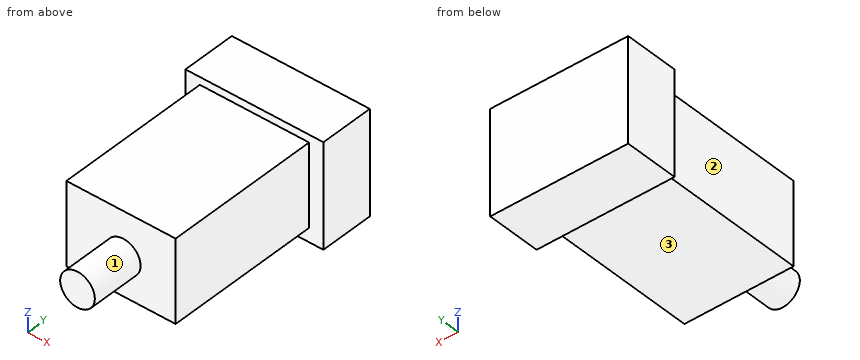
```python
from build123d import *

# Parameters (mm, degrees)
F0_W     = 101.638708
F0_H     = 76.456577
F1_DEPTH = 39.878
F2_W     = 80.470148
F2_H     = 60.710575
F3_DEPTH = 114.808
F4_R     = 12.763073
F5_DEPTH = 39.37
F6_W     = 52.336872
F6_H     = 92.136786
F7_DEPTH = 27.94


with BuildPart() as f1:
    # F0 (on Front) → F1 (new body)
    with BuildSketch(Plane.XZ):
        with Locations((-1.668697, -0.151697)):
            Rectangle(F0_W, F0_H)
    extrude(amount=F1_DEPTH)

    # F2 (on face) → F3 (join)
    with BuildSketch(Plane.XZ.offset(39.878)):
        with Locations((-1.668697, 2.139264)):
            Rectangle(F2_W, F2_H)
    extrude(amount=F3_DEPTH)

    # F4 (on face) → F5 (join)
    with BuildSketch(Plane.XZ.offset(154.686)):
        Circle(F4_R)
    extrude(amount=F5_DEPTH)

    # F6 (on face) → F7 (join)
    with BuildSketch(Plane.XY.offset(32.494552)):
        with Locations((-0.389457, -95.996715)):
            Rectangle(F6_W, F6_H)
    extrude(amount=-F7_DEPTH)


solid = f1.part
```
Input: part model. Units: mm. Frame: model coordinates. Face numbers are marked on the shaded views. A direction names the side the tool comes from. Coordinates: 2 decimals unless noted, no trailing zeros. Write each loop counter-clockwise with the first axis right and the second up, starting at its lowest first coordinate (ties: lowest second). Pieces come first, ordered by that corner, then holes. Notation, with made-up numbers: (85.5, 16.5) -> (98.5, 16.5) arc R17 cw to (98.5, 23.5) -> close; hole circle Ø1 at (-18, -32.5). An arc over 180 degrees is marked (long way). Answer as a JSON object with one key per item and string values.
1. Section C-C on y = -42.5. Return the cut outline in (x, z), then the cut area to 3 significant figures.
Result set:
{"outline": "(-41.9, -28.22) -> (38.57, -28.22) -> (38.57, 32.49) -> (-41.9, 32.49) -> close", "area": "4,890 mm2"}
2. Section D-D on z = -19.5. Return the cut outline in (x, y).
Result set:
{"outline": "(-52.49, -39.88) -> (-41.9, -39.88) -> (-41.9, -154.69) -> (38.57, -154.69) -> (38.57, -39.88) -> (49.15, -39.88) -> (49.15, 0) -> (-52.49, 0) -> close"}
3. First-contact query: P1, Ø1.5, axis at x = -2.5, y = -69, coming from the -Z side; P2, Ø18, axis at y = -72.5, z = 10.5, coming from the -X side; P3, Ø5, axis at x = -22.5, y = -135, coming from the +Z side; P4, Ø1, axis at y = -102.5, z = -29.5, coming from the -X side. Flat tips, straight axial feed; report the tip coordinate or a pass-through.
Result set:
{"P1": "stops at z = -28.22", "P2": "stops at x = -41.9", "P3": "stops at z = 32.49", "P4": "passes through"}
4. Material intervals for line 1 (Y direction, x = -20.5, z = 33); line 2 (X direction, y = -75.5, z = -7.5); line 3 (Y direction, x = -12, z = 13), sorted ascending. Write a range as from..to.
Result set:
{"line 1": "y = -39.88..0", "line 2": "x = -41.9..38.57", "line 3": "y = -154.69..0"}
5. Access query for the marked faces 1, 2 and 3. Directions: +Z, -Z, +X, -X, +Y, -Y. A direction counts if a zero-diameter tool reaches every point of the face in a straight line with its end or side. Return the directions, or none.
Result set:
{"face 1": "-Y", "face 2": "+Z, -Z, -X, -Y", "face 3": "-Z, +X, -X, -Y"}
6. Section A-A on z = 0. Return the cut outline in (x, y), then the cut area to 3 significant figures.
Result set:
{"outline": "(-52.49, -39.88) -> (-41.9, -39.88) -> (-41.9, -154.69) -> (-12.76, -154.69) -> (-12.76, -194.06) -> (12.76, -194.06) -> (12.76, -154.69) -> (38.57, -154.69) -> (38.57, -39.88) -> (49.15, -39.88) -> (49.15, 0) -> (-52.49, 0) -> close", "area": "14,300 mm2"}
7. Section B-B on x = 0. Return the cut outline in (y, z).
Result set:
{"outline": "(-194.06, -12.76) -> (-154.69, -12.76) -> (-154.69, -28.22) -> (-39.88, -28.22) -> (-39.88, -38.38) -> (0, -38.38) -> (0, 38.08) -> (-39.88, 38.08) -> (-39.88, 32.49) -> (-154.69, 32.49) -> (-154.69, 12.76) -> (-194.06, 12.76) -> close"}
